from build123d import *

# Parameters (mm, degrees)
SKETCH_1_R          = 500
EXTRUDE_1_DEPTH     = 50
SKETCH_2_W          = 50
SKETCH_2_H          = 50
EXTRUDE_2_DEPTH     = 700
SKETCH_3_W          = 50
SKETCH_3_H          = 50
EXTRUDE_3_DEPTH     = 700
SKETCH_4_W          = 50
SKETCH_4_H          = 50
EXTRUDE_4_DEPTH     = 700
SKETCH_5_W          = 50
SKETCH_5_H          = 50
EXTRUDE_5_DEPTH     = 700
SKETCH_6_W          = 200
SKETCH_6_H          = 100
EXTRUDE_6_DEPTH     = 50
SKETCH_7_W          = 150
SKETCH_7_H          = 50
CUT_EXTRUDE_1_DEPTH = 30


with BuildPart() as part:
    # 草图1 → 凸台-拉伸1 (new body)
    with BuildSketch(Plane.XY):
        Circle(SKETCH_1_R)
    extrude(amount=EXTRUDE_1_DEPTH)

    # 草图2 → 凸台-拉伸2 (add)
    with BuildSketch(Plane.XY):
        with Locations((250, 250)):
            Rectangle(SKETCH_2_W, SKETCH_2_H)
    extrude(amount=EXTRUDE_2_DEPTH)

    # 草图3 → 凸台-拉伸3 (add)
    with BuildSketch(Plane.XY):
        with Locations((-250, 250)):
            Rectangle(SKETCH_3_W, SKETCH_3_H)
    extrude(amount=EXTRUDE_3_DEPTH)

    # 草图4 → 凸台-拉伸4 (add)
    with BuildSketch(Plane.XY):
        with Locations((250, -250)):
            Rectangle(SKETCH_4_W, SKETCH_4_H)
    extrude(amount=EXTRUDE_4_DEPTH)

    # 草图5 → 凸台-拉伸5 (add)
    with BuildSketch(Plane.XY):
        with Locations((-250, -250)):
            Rectangle(SKETCH_5_W, SKETCH_5_H)
    extrude(amount=EXTRUDE_5_DEPTH)

    # 草图6 → 凸台-拉伸6 (add)
    with BuildSketch(Plane(origin=(0, 275, 0), x_dir=(1, 0, 0), z_dir=(0, 1, 0))):
        Rectangle(SKETCH_6_W, SKETCH_6_H)
    extrude(amount=EXTRUDE_6_DEPTH)

    # 草图7 → 切除-拉伸1 (cut)
    with BuildSketch(Plane(origin=(0, 275, 0), x_dir=(1, 0, 0), z_dir=(0, 1, 0))):
        Rectangle(SKETCH_7_W, SKETCH_7_H)
    extrude(amount=CUT_EXTRUDE_1_DEPTH, mode=Mode.SUBTRACT)


solid = part.part
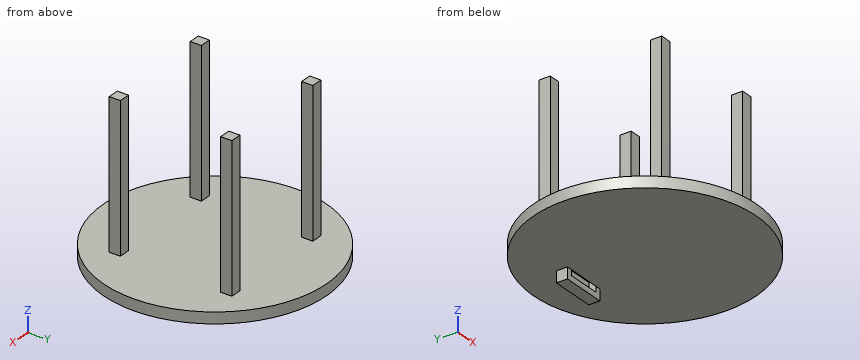
Geometry: final body of the model. Coordinates: model frame, mm. Give positions to 0.01 mm unless a question says otherwise; leave off trailing zeros. Loops run counter-clockwise (first coordinate to the right, second up) from the corner with the lowest first, then second, coordinate; pieces in that order, holes last. Notation, with made-up numbers: (71, 11.25) - (82, 11.25) arc R20 ccw to (82, 29.25) - close; hole circle Ø8 at (9, 27.5). An arc over 180 degrees is marked (long way). Answer as CSV lines item,"result". Start each with the question number.
1. Section B-B, the plane x = 0. Return loops of the section in (y, z).
2. Section D-D, the plane y = 0. Return loops of the section in (x, z).
3. Ray query, L1, parallel to Y at x = 252, z = 299.5; L2, parallel to Z at x = 139.5, y = 51.5; L3, parallel to Z at x = 99, y = 308. Return the intervals inside material, ascending.
4. Section C-C, the plane y = -261. Return loops of the section in (x, z).
5. Section A-A, the plane z = 367.5. Return loops of the section in (x, y), plus the area to 3 significant figures.
6. Pin query (flat end, axial travel): P1, Ø24, axis at x = 17.5, y = 296.5, coming from the +Z side; P2, Ø2, axis at x = -104, y = -389.5, coming from the -Z side; P3, Ø15, axis at x = -42, z = -25, coming from the -Y side. Return the tip coordinate at first contact, or that it passes through.
Answers:
1,outline,"(-500, 0) - (275, 0) - (275, 25) - (305, 25) - (305, -25) - (275, -25) - (275, -50) - (325, -50) - (325, 0) - (500, 0) - (500, 50) - (-500, 50) - close"
2,outline,"(-500, 0) - (500, 0) - (500, 50) - (-500, 50) - close"
3,L1,"y = -275 to -225, 225 to 275"
3,L2,"z = 0 to 50"
3,L3,"z = -50 to 50"
4,outline,"(-426.47, 0) - (426.47, 0) - (426.47, 50) - (275, 50) - (275, 700) - (225, 700) - (225, 50) - (-225, 50) - (-225, 700) - (-275, 700) - (-275, 50) - (-426.47, 50) - close"
5,outline,"(-275, -275) - (-225, -275) - (-225, -225) - (-275, -225) - close; (-275, 225) - (-225, 225) - (-225, 275) - (-275, 275) - close; (225, -275) - (275, -275) - (275, -225) - (225, -225) - close; (225, 225) - (275, 225) - (275, 275) - (225, 275) - close"
5,area,"10,000 mm2"
6,P1,"stops at z = 50"
6,P2,"stops at z = 0"
6,P3,"stops at y = 275"
